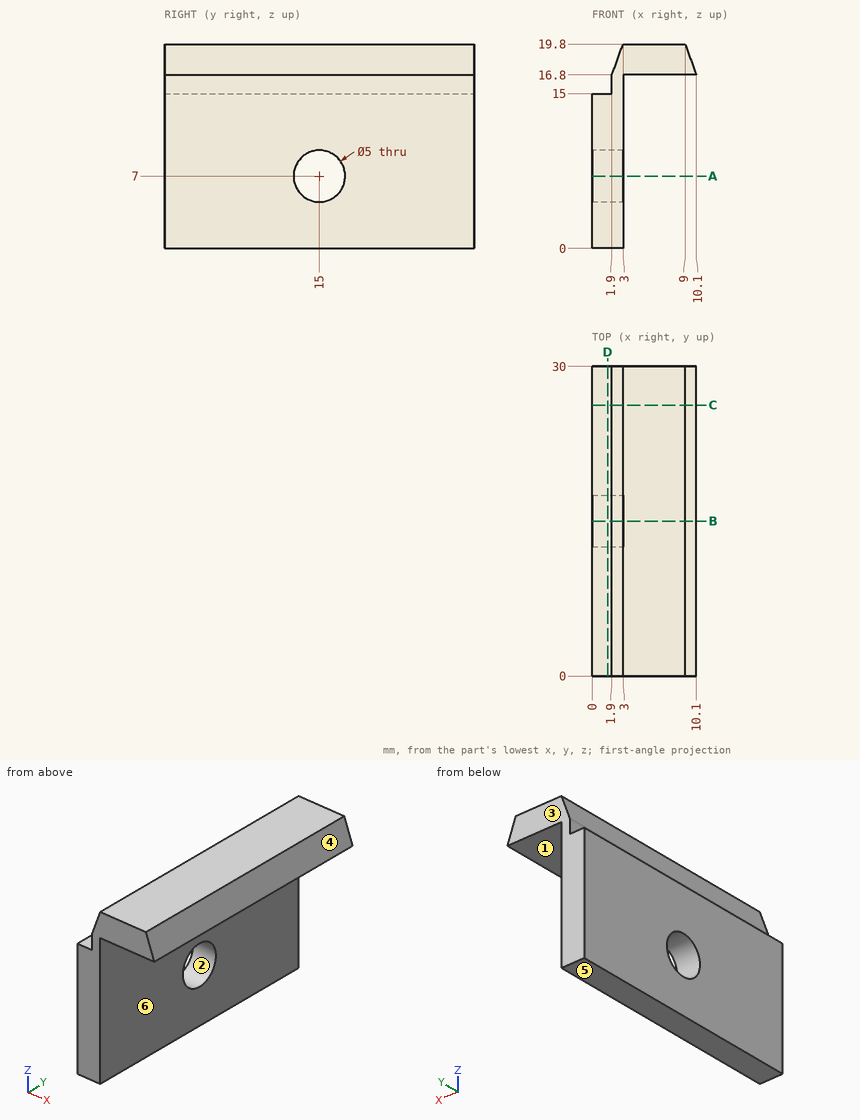
Here's the drawing with two shaded views (mm, measured from the low corner). I have some questions. A direction names the side the tool comes from. Coordinates: 2 decimals unless noted, no trailing zeros. Write each loop counter-clockwise with the first axis right and the second up, starting at its lowest first coordinate (ties: lowest second). Pieces come first, ordered by that corner, then holes. Notation, with made-up numbers: (73, 1) -> (113, 1) arc R13 ccw to (113, 25) -> close; hole circle Ø6 at (-8, 69). An arc over 180 degrees is marked (long way). Write item = value, one per line. Start each with the question number.
(1) Which directions (+Z, -Z, +X, -X, +Y, -Y) give clear straight access to the entire face, cutting with the end or side of a thin tool? Please do the marked faces 5 and 6.
(2) We'd pull the mould along Z, two halves only. Please class the marked faces 1, 2, 3 and 4: released by +Z, released by -Z, zero draft, split by the parting line, or undercut.
(3) I want a section at D-D (x = 1.5). Please give me the cut outline in (y, z).
(4) I need wall thicknesses on line 1 (Z direction, x = 1.85, y = 15); line 2 (Y direction, x = 0.8, z = 7); line 3 (Z direction, x = 4.5, y = 25). Which ranges of each line are inside material? Lowest first, please. Write a range as [from, to].
(5) Will these pins go through, and if not, where does the flat tip stop? pin 1 (1.4 mm diameter, centred on y = 7.5, z = 16, fed in from -X); pin 2 (2 mm diameter, centred on y = 16.5, z = 14.5, fed in from +X); pin 3 (1 mm diameter, centred on x = 0.5, y = 15.5, fed in from +Z).
(6) I want a section at C-C (y = 26.25). Please give me the cut outline in (x, z), plus the area to 3 significant figures.
(7) I want a section at B-B (y = 15). Please give me the cut outline in (x, z), plus the area to 3 significant figures.
(8) I want a section at A-A (z = 7). Please give me the cut outline in (x, y).
Result set:
q1.face_5 = -Z, +X, -X, +Y, -Y
q1.face_6 = -Z, +X, +Y, -Y
q2.face_1 = released by -Z
q2.face_2 = undercut
q2.face_3 = zero draft
q2.face_4 = released by +Z
q3.outline = (0, 0) -> (30, 0) -> (30, 15) -> (0, 15) -> close; hole circle Ø5 at (15, 7)
q4.line_1 = [0, 4.5], [9.5, 15]
q4.line_2 = [0, 12.5], [17.5, 30]
q4.line_3 = [16.8, 19.8]
q5.pin_1 = 1.9
q5.pin_2 = 3
q5.pin_3 = 15
q6.outline = (0, 0) -> (3, 0) -> (3, 16.8) -> (10.1, 16.8) -> (9, 19.8) -> (3, 19.8) -> (1.9, 16.8) -> (1.9, 15) -> (0, 15) -> close
q6.area = 68.3 mm2
q7.outline = (0, 0) -> (3, 0) -> (3, 4.5) -> (0, 4.5) -> close; (0, 9.5) -> (3, 9.5) -> (3, 16.8) -> (10.1, 16.8) -> (9, 19.8) -> (3, 19.8) -> (1.9, 16.8) -> (1.9, 15) -> (0, 15) -> close
q7.area = 53.3 mm2
q8.outline = (0, 0) -> (3, 0) -> (3, 12.5) -> (0, 12.5) -> close; (0, 17.5) -> (3, 17.5) -> (3, 30) -> (0, 30) -> close
